Build history of the part. All positions in model axes, mm. Round coordinates to 2 decimals unless told otherwise and drop trailing zeros. Write each loop counter-clockwise with the first axis right and the second up, starting at its lowest first coordinate (ties: lowest second). Pieces come first, ordered by that corner, then holes.
Item 1: Wall check: probe 1 along Y at (x, z) = (37, 0.45) (3 decimals); probe 2 along X at (y, z) = (-3.75, 0.35); probe 3 along X at (y, z) = (-2.25, 0.85). Give the ranges that are in metal, low to high.
Item 2: Band-saw the part on D-D, the plane x = -5. Write the cut outline in (y, z) (3 decimals).
Item 3: Band-saw the part on A-A, the plane y = 1.75. Write the cut outline in (x, z), then the cut area to 3 significant figures.
Item 4: Drop a flat-ended pin along its axis: pin 1 Ø1 at (x, z) = (-13.5, 1) entering from +Y (3 decimals). Give the stop position or say it passes through.
Item 5: Band-saw the part on B-B, the plane x = -38. Write the cut outline in (y, z) (3 decimals), then the cut area to 3 significant figures.
Item 6: Band-saw the part on C-C, the plane z = 0.85. Write the cut outline in (x, y) (3 decimals), then the cut area to 3 significant figures.
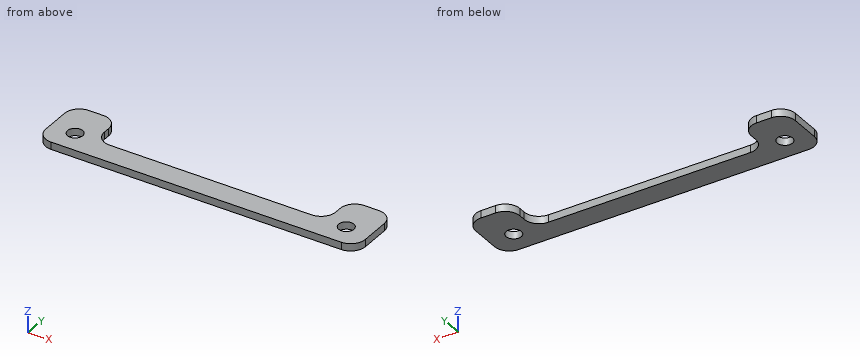
```python
from build123d import *

# Parameters (mm, degrees)
F0_R     = 2.074641
F1_DEPTH = 2


with BuildPart() as f1:
    # F0 (on Top) → F1 (new body)
    with BuildSketch(Plane.XY):
        with BuildLine():
            Line((-39.5, -9.535), (39.5, -9.535))
            ThreePointArc((39.5, -9.535), (42.328427, -8.363427), (43.5, -5.535))
            Line((43.5, -5.535), (43.5, 2.465))
            ThreePointArc((43.5, 2.465), (42.328427, 5.293427), (39.5, 6.465))
            Line((39.5, 6.465), (35.5, 6.465))
            ThreePointArc((35.5, 6.465), (32.671573, 5.293427), (31.5, 2.465))
            Line((31.5, 2.465), (31.5, 0.605))
            ThreePointArc((31.5, 0.605), (30.328427, -2.223427), (27.5, -3.395))
            Line((27.5, -3.395), (-27.5, -3.395))
            ThreePointArc((-27.5, -3.395), (-30.328427, -2.223427), (-31.5, 0.605))
            Line((-31.5, 0.605), (-31.5, 2.465))
            ThreePointArc((-31.5, 2.465), (-32.671573, 5.293427), (-35.5, 6.465))
            Line((-35.5, 6.465), (-39.5, 6.465))
            ThreePointArc((-39.5, 6.465), (-42.328427, 5.293427), (-43.5, 2.465))
            Line((-43.5, 2.465), (-43.5, -5.535))
            ThreePointArc((-43.5, -5.535), (-42.328427, -8.363427), (-39.5, -9.535))
        make_face()
        with Locations((-36.891578, -3.354191)):
            Circle(F0_R, mode=Mode.SUBTRACT)
        with Locations((36.891578, -3.354191)):
            Circle(F0_R, mode=Mode.SUBTRACT)
    extrude(amount=F1_DEPTH)


solid = f1.part
```
Results:
1. probe 1: y = -9.535 to -5.426, -1.282 to 6.465
1. probe 2: x = -43.5 to -38.93, -34.86 to 34.86, 38.93 to 43.5
1. probe 3: x = -43.5 to -38.65, -35.14 to -30.3, 30.3 to 35.14, 38.65 to 43.5
2. outline: (-9.535, 0) - (-3.395, 0) - (-3.395, 2) - (-9.535, 2) - close
3. outline: (-43.5, 0) - (-31.5, 0) - (-31.5, 2) - (-43.5, 2) - close; (31.5, 0) - (43.5, 0) - (43.5, 2) - (31.5, 2) - close
3. area: 48.0 mm2
4. pin 1: stops at y = -3.395
5. outline: (-9.535, 0) - (-5.108, 0) - (-5.108, 2) - (-9.535, 2) - close; (-1.6, 0) - (6.465, 0) - (6.465, 2) - (-1.6, 2) - close
5. area: 25.0 mm2
6. outline: (-43.5, -5.535) arc R4 ccw to (-39.5, -9.535) - (39.5, -9.535) arc R4 ccw to (43.5, -5.535) - (43.5, 2.465) arc R4 ccw to (39.5, 6.465) - (35.5, 6.465) arc R4 ccw to (31.5, 2.465) - (31.5, 0.605) arc R4 cw to (27.5, -3.395) - (-27.5, -3.395) arc R4 cw to (-31.5, 0.605) - (-31.5, 2.465) arc R4 ccw to (-35.5, 6.465) - (-39.5, 6.465) arc R4 ccw to (-43.5, 2.465) - close; hole circle Ø4.149 at (-36.892, -3.354); hole circle Ø4.149 at (36.892, -3.354)
6. area: 730 mm2
